```python
from build123d import *

# Parameters (mm, degrees)
SKETCH2_W           = 25.4
SKETCH2_H           = 403.225
BOSS_EXTRUDE1_DEPTH = 3.175
SKETCH3_W           = 8.466666666
SKETCH3_H           = 3.175
CUT_EXTRUDE1_DEPTH  = 3.175
CUT_EXTRUDE2_DEPTH  = 3.175


with BuildPart() as part:
    # Sketch2 → Boss-Extrude1 (new body)
    with BuildSketch(Plane(origin=(0, 0, 0), x_dir=(1, 0, 0), z_dir=(0, 1, 0))):
        Rectangle(SKETCH2_W, SKETCH2_H)
    extrude(amount=BOSS_EXTRUDE1_DEPTH)

    # Sketch3 → Cut-Extrude1 (cut)
    with BuildSketch(Plane(origin=(0, 3.175, 0), x_dir=(1, 0, 0), z_dir=(0, 1, 0))):
        with Locations((0, 200.025)):
            Rectangle(SKETCH3_W, SKETCH3_H)
    cut_extrude1 = extrude(amount=-CUT_EXTRUDE1_DEPTH, mode=Mode.SUBTRACT)

    # Mirror1: Cut-Extrude1 across plane
    add(cut_extrude1.mirror(Plane.XY), mode=Mode.SUBTRACT)

    # Sketch5 → Cut-Extrude2 (cut)
    with BuildSketch(Plane(origin=(0, 3.175, 0), x_dir=(1, 0, 0), z_dir=(0, 1, 0))):
        with BuildLine():
            ThreePointArc((8.217514421, -83.769985579), (6.717514421, -82.269985579), (5.217514421, -83.769985579))
            Line((5.217514421, -83.769985579), (6.717514421, -83.769985579))
            Line((6.717514421, -83.769985579), (6.717514421, -85.269985579))
            ThreePointArc((6.717514421, -85.269985579), (7.778174593, -84.830645751), (8.217514421, -83.769985579))
        make_face()
        with BuildLine():
            Line((6.717514421, -83.769985579), (5.217514421, -83.769985579))
            ThreePointArc((5.217514421, -83.769985579), (5.656854249, -84.830645751), (6.717514421, -85.269985579))
            Line((6.717514421, -85.269985579), (6.717514421, -83.769985579))
        make_face()
        with BuildLine():
            Line((-6.717514421, -85.269985579), (-6.717514421, -83.769985579))
            Line((-6.717514421, -83.769985579), (-5.217514421, -83.769985579))
            ThreePointArc((-5.217514421, -83.769985579), (-7.778174593, -82.709325407), (-6.717514421, -85.269985579))
        make_face()
        with BuildLine():
            Line((-5.217514421, -83.769985579), (-6.717514421, -83.769985579))
            Line((-6.717514421, -83.769985579), (-6.717514421, -85.269985579))
            ThreePointArc((-6.717514421, -85.269985579), (-5.656854249, -84.830645751), (-5.217514421, -83.769985579))
        make_face()
        with BuildLine():
            ThreePointArc((-5.217514421, -97.205014421), (-5.656854249, -96.144354249), (-6.717514421, -95.705014421))
            Line((-6.717514421, -95.705014421), (-6.717514421, -97.205014421))
            Line((-6.717514421, -97.205014421), (-5.217514421, -97.205014421))
        make_face()
        with BuildLine():
            Line((-6.717514421, -97.205014421), (-6.717514421, -95.705014421))
            ThreePointArc((-6.717514421, -95.705014421), (-7.778174593, -98.265674593), (-5.217514421, -97.205014421))
            Line((-5.217514421, -97.205014421), (-6.717514421, -97.205014421))
        make_face()
        with BuildLine():
            ThreePointArc((8.217514421, -97.205014421), (7.778174593, -96.144354249), (6.717514421, -95.705014421))
            Line((6.717514421, -95.705014421), (6.717514421, -97.205014421))
            Line((6.717514421, -97.205014421), (5.217514421, -97.205014421))
            ThreePointArc((5.217514421, -97.205014421), (6.717514421, -98.705014421), (8.217514421, -97.205014421))
        make_face()
        with BuildLine():
            Line((6.717514421, -97.205014421), (6.717514421, -95.705014421))
            ThreePointArc((6.717514421, -95.705014421), (5.656854249, -96.144354249), (5.217514421, -97.205014421))
            Line((5.217514421, -97.205014421), (6.717514421, -97.205014421))
        make_face()
    cut_extrude2 = extrude(amount=-CUT_EXTRUDE2_DEPTH, mode=Mode.SUBTRACT)

    # Mirror2: Cut-Extrude2 across plane
    add(cut_extrude2.mirror(Plane.XY), mode=Mode.SUBTRACT)


solid = part.part
```
Read the model definition and answer for the solid it produces. Units are mm, in the model's axes. Coordinates: 2 decimals unless noted, no trailing zeros. Loops run counter-clockwise (first coordinate to the right, second up) from the corner with the lowest first, then second, coordinate; pieces in that order, holes last.
(1) Flat-ended cylindrical pins translate along their axes: pin 1 Ø1.6 at (x, y) = (2, 1.5) entering from -Z; pin 2 Ø1.8 at (x, z) = (-6.72, 83.77) entering from +Y. Find the tip coordinate at first contact, or state that the pin passes through.
Solution:
pin 1: stops at z = -198.44
pin 2: passes through
(2) Consider line 1 along X through (y, z) = (2.2, 97.5); line 2 along Z through (x, y) = (6.75, 2.35); line 3 along Z through (x, y) = (6, 2.8). Determine where each line is inside the solid, lowest interval first.
Solution:
line 1: x = -12.7 to -8.19, -5.25 to 5.25, 8.19 to 12.7
line 2: z = -201.61 to -98.7, -95.71 to -85.27, -82.27 to 82.27, 85.27 to 95.71, 98.7 to 201.61
line 3: z = -201.61 to -98.52, -95.89 to -85.09, -82.45 to 82.45, 85.09 to 95.89, 98.52 to 201.61
(3) The part is cut by section A-A (x = 1). Determine the outline of the cut face in (y, z) (1 decimal), and give its area (3 significant figures).
Solution:
outline: (0, -198.4) - (3.2, -198.4) - (3.2, 198.4) - (0, 198.4) - close
area: 1,260 mm2
